Part print with two shaded views. Sizes in mm from the minimum x, y, z corner. A direction names the side the tool comes from. Give positions to 0.01 mm unless a question says otherwise; leave off trailing zeros. Write each loop counter-clockwise with the first axis right and the second up, starting at its lowest first coordinate (ties: lowest second). Pieces come first, ordered by that corner, then holes. Notation, with made-up numbers: (80.25, 53.25) -> (120.25, 53.25) arc R34 cw to (120.25, 91.25) -> close; hole circle Ø10 at (86, -11). An arc over 180 degrees is marked (long way). Write item = value, one per line. Start each with the question number.
Q1. Saw through at A-A, the plane z = 15. List the corners of the cut face in (x, y).
Q2. Saw through at D-D, the plane z = 9.25. List the corners of the cut face in (x, y) (1 decimal).
Q3. Drop flat-ended pins along their axis: P1, Ø1.2, axis at x = 1, z = 14.5, coming from the -Y side; P2, Ø0.5, axis at x = 1.5, z = 12.5, coming from the +Y side (1 decimal); P3, Ø1, axis at x = 1, y = 4, coming from the -Z side (1 decimal). Give the stop position or say it passes through.
Q4. Saw through at C-C, the plane y = 3.5. List the corners of the cut face in (x, z) (1 decimal).
Q5. Wall check: line 1 (Y direction, x = 1.1, z = 16.5) (1 decimal); line 2 (Z direction, x = 2.3, y = 8.5) (1 decimal); line 3 (Y direction, x = 1.95, z = 13.5). Give the ranges that are in metal, low to high.
Q6. Tool access for the marked faces 1 and 2: list every direction of +Z, -Z, +X, -X, +Y, -Y with a clear straight run to the whole face (end or side of a thin tool).
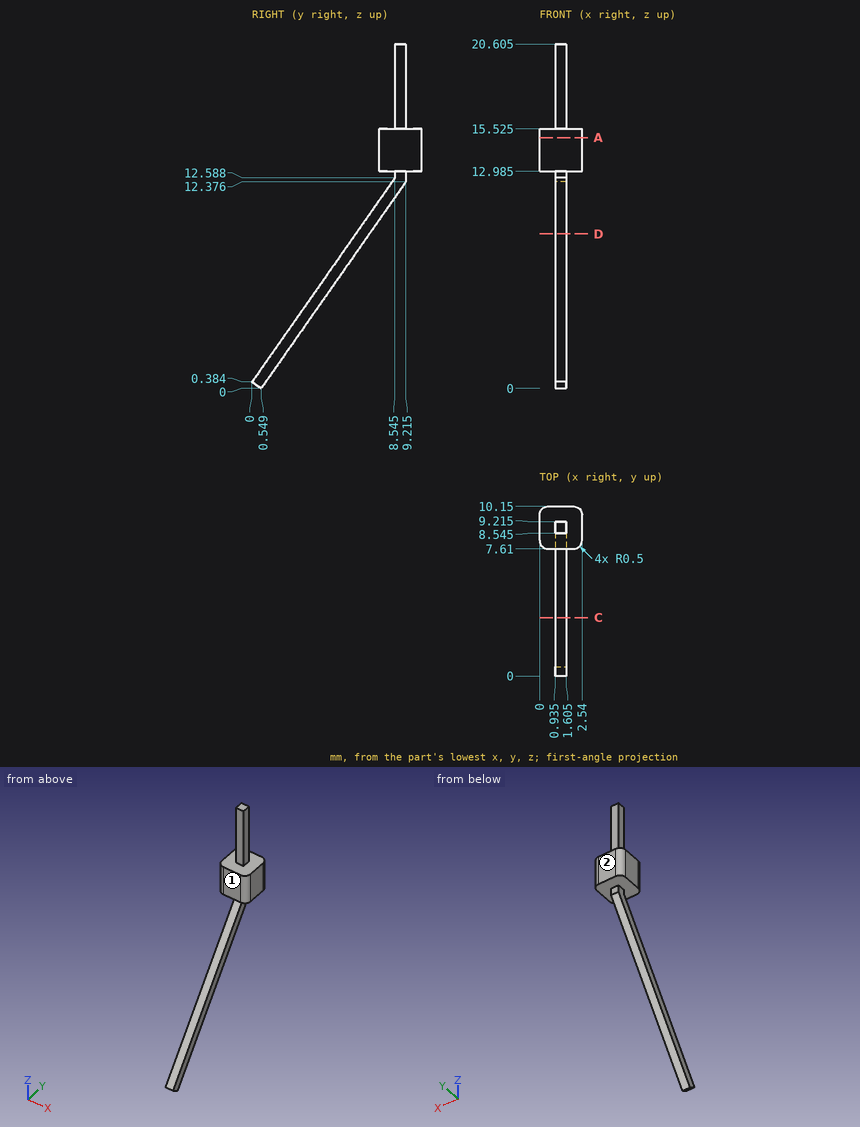
Report:
q1.outline = (0, 8.11) arc R0.5 ccw to (0.5, 7.61) -> (2.04, 7.61) arc R0.5 ccw to (2.54, 8.11) -> (2.54, 9.65) arc R0.5 ccw to (2.04, 10.15) -> (0.5, 10.15) arc R0.5 ccw to (0, 9.65) -> close
q2.outline = (0.9, 6.2) -> (1.6, 6.2) -> (1.6, 7) -> (0.9, 7) -> close
q3.P1 = 7.61
q3.P2 = 9.2
q3.P3 = 4.2
q4.outline = (0.9, 4.2) -> (1.6, 4.2) -> (1.6, 5.4) -> (0.9, 5.4) -> close
q5.line_1 = 8.5 to 9.2
q5.line_2 = 13 to 15.5
q5.line_3 = 7.61 to 10.15
q6.face_1 = +Z, +X, -X, -Y
q6.face_2 = +Z, -Z, +X, -X, +Y
